Read the model definition and answer for the solid it produces. Units are mm, in the model's axes. A direction names the side the tool comes from. Round coordinates to 2 decimals unless told otherwise and drop trailing zeros. Write each loop counter-clockwise with the first axis right and the second up, starting at its lowest first coordinate (ties: lowest second). Pieces come first, ordered by that corner, then holes. Notation, with made-up numbers: (14.5, 27) -> (31.5, 27) arc R31 ccw to (31.5, 60) -> close; hole circle Ø5 at (7, 60). An arc over 180 degrees is marked (long way). Return JSON: item names as keys, results as strings. Group by question number.
(1) A cutting plane is placed at A-A on z = 15. Give the vertices of the cut face in (x, y), then the cut area to 3 significant figures.
(2) Straight lines are drawn through the part: line 1 (Z direction, x = 8, y = 1.25); line 2 (X direction, y = 2.25, z = 13.5); line 3 (Y direction, x = 4.75, z = 14.5). For each, find the intervals that lie inside material, in ascending order.
(3) A cutting plane is placed at C-C on y = 1. Give the vertices of the cut face in (x, z).
(4) A cutting plane is placed at B-B on z = 5. Give the vertices of the cut face in (x, y), then the cut area to 3 significant figures.
(5) Given pin 1 (3.5 mm diameter, centred on x = 7, z = 14.5, fed in from +Y); pin 2 (3.5 mm diameter, centred on x = 9.5, z = 14.5, fed in from -Y); pin 3 (2 mm diameter, centred on x = 9.5, z = 4.5, fed in from -Y), each flat-ended and moving along its own axis, determine where each tip first touches the part or whether it passes through.
(6) A cutting plane is placed at D-D on x = 1.5. Give the vertices of the cut face in (y, z) (3 decimals).
(7) The mould has two halves that part along X. Classify faces 1 (the flat face through (6.9, 4.5, -8.5)), 2 (the flat face through (6.9, 2, -6.5)), 3 (the flat face through (4, 3.5, -7.7)): released by +X, released by -X, zero draft, split by the parting line, or undercut.
(8) For faces 4 (the flat face through (9, 1, -5)), 5 (the flat face through (7, 1, -6)), 6 (the flat face through (6.9, 4.5, -6.5)), 7 (the flat face through (1.2, 3, 17)), 8 (the flat face through (7, 1.5, 17)), determine the directions among +Z, -Z, +X, -X, +Y, -Y from which every point of the face is accessible in a straight line to the end or side of a thin tool.
Autodesk Fusion 360 part; units mm, degrees
sketch "草图1" plane through (0, 0, 0) normal (0, 1, 0) x (1, 0, 0)
  line L0 (0, 0) -> (14, 0)
  line L1 (14, 0) -> (14, -11)
  line L2 (14, -11) -> (0, -11)
  line L3 (0, -11) -> (0, 0)
  line L4 (7, -11) -> (7, 8) construction
  line L5 (7, 5) -> (10, 5)
  line L6 (7, 5) -> (4, 5)
  line L7 (0, 0) -> (4, 5)
  line L8 (14, 0) -> (10, 5)
  dimension "d1" = 14
  dimension "d2" = 11
  dimension "d3" = 3
  dimension "d4" = 3
  dimension "d5" = 5
extrude "拉伸1" add sketch "草图1" along normal blind 7
sketch "草图2" plane through (0, 0, 11) normal (0, 0, 1) x (-1, 0, 0)
  line L0 (0, 0) -> (-14, 0)
  line L1 (-14, 0) -> (-14, -7)
  line L2 (-14, -7) -> (0, -7)
  line L3 (0, -7) -> (0, 0)
  line L4 (-1, -5.5) -> (-13, -5.5)
  line L5 (-13, -5.5) -> (-13, -1.5)
  line L6 (-13, -1.5) -> (-1, -1.5)
  line L7 (-1, -1.5) -> (-1, -5.5)
  line L8 (-1.2, -1.7) -> (-1.2, -5.3)
  line L9 (-1.2, -5.3) -> (-12.8, -5.3)
  line L10 (-12.8, -5.3) -> (-12.8, -1.7)
  line L11 (-12.8, -1.7) -> (-1.2, -1.7)
  line L12 (-1.2, -3.5) -> (-12.8, -3.5)
  dimension "d8" = 12
  dimension "d9" = 4
  dimension "d10" = 1.5
  dimension "d11" = 1
  dimension "d12" = 0.2
extrude "拉伸2" add sketch "草图2" along normal blind 12 contours L4 L5 L6 L7
extrude "拉伸3" add sketch "草图2" along normal blind 11 contours L8 L9 L10 L12
sketch "草图3" plane through (0, 0, 0) normal (0, -1, 0) x (1, 0, 0)
  line L0 (14, 0) -> (14, 11)
  line L1 (14, 11) -> (0, 11)
  line L2 (0, 11) -> (0, 0)
  line L3 (0, 0) -> (4, -5)
  line L4 (4, -5) -> (10, -5)
  line L5 (10, -5) -> (14, 0)
  line L6 (2, 9) -> (12, 9)
  line L7 (12, 9) -> (12, 0)
  line L8 (12, 0) -> (2, 0)
  line L9 (2, 0) -> (2, 9)
extrude "拉伸4" cut sketch "草图3" against normal blind 0.2 contours L6 L7 L8 L9
sketch "草图4" plane through (0, 7, 0) normal (0, 1, 0) x (-1, 0, 0)
  line L0 (-14, 11) -> (-14, 0)
  line L1 (-14, 0) -> (-10, -5)
  line L2 (-10, -5) -> (-4, -5)
  line L3 (-4, -5) -> (0, 0)
  line L4 (0, 0) -> (0, 11)
  line L5 (0, 11) -> (-14, 11)
  line L6 (-12, 9) -> (-2, 9)
  line L7 (-2, 9) -> (-2, 0)
  line L8 (-2, 0) -> (-12, 0)
  line L9 (-12, 0) -> (-12, 9)
extrude "拉伸5" cut sketch "草图4" against normal blind 0.2 contours L6 L7 L8 L9
sketch "草图5" plane through (0, 1.5, 0) normal (0, -1, 0) x (1, 0, 0)
  line L0 (1, 11) -> (13, 11)
  line L1 (13, 11) -> (13, 23)
  line L2 (13, 23) -> (1, 23)
  line L3 (1, 23) -> (1, 11)
  line L4 (7, 11) -> (7, 23) construction
  line L5 (2.5, 20) -> (5.5, 20)
  line L6 (5.5, 20) -> (5.5, 18)
  line L7 (5.5, 18) -> (2.5, 18)
  line L8 (2.5, 18) -> (2.5, 20)
  line L9 (11.5, 20) -> (8.5, 20)
  line L10 (11.5, 18) -> (11.5, 20)
  line L11 (8.5, 18) -> (11.5, 18)
  line L12 (8.5, 20) -> (8.5, 18)
  dimension "d21" = 1.5
extrude "拉伸6" cut sketch "草图5" against normal up to surface (0.2 mm away) contours L5 L6 L7 L8 | L9 L10 L11 L12
sketch "草图6" plane through (0, 0, -5) normal (0, 0, -1) x (1, 0, 0)
  line L0 (10, 0) -> (4, 0)
  line L1 (4, 0) -> (4, -7)
  line L2 (4, -7) -> (10, -7)
  line L3 (10, -7) -> (10, 0)
  circle A0 centre (6.9717, -3.5) radius 3
  dimension "d24" = 6
extrude "拉伸7" add sketch "草图6" along normal blind 5.5 contours L1 A0 picked at (7.5942, -2.8884)
sketch "草图7" plane through (0, 0, 0) normal (0, 1, 0) x (1, 0, 0)
  line L0 (4, 6) -> (10, 6)
  line L1 (10, 6) -> (10, 7)
  line L2 (10, 7) -> (4, 7)
  line L3 (4, 7) -> (4, 6)
  line L4 (4, 8) -> (10, 8)
  line L5 (10, 8) -> (10, 9)
  line L6 (10, 9) -> (4, 9)
  line L7 (4, 9) -> (4, 8)
extrude "拉伸8" cut sketch "草图7" along normal blind 2
extrude "拉伸9" cut 2 faces at (6.1056, 2, -6.3333) (6.1056, 2, -8.3333) along direction (0, 1, 0) blind 2 from surface at 2.5
Checks:
{
 "1": {"outline": "(1, 1.5) -> (13, 1.5) -> (13, 5.5) -> (1, 5.5) -> close; hole (1.2, 1.7) -> (12.8, 1.7) -> (12.8, 3.5) -> (1.2, 3.5) -> close", "area": "27.1 mm^2"},
 "2": {"line 1": "z = -10.5 to -9, -8 to -7, -6 to 11", "line 2": "x = 1 to 1.2, 12.8 to 13", "line 3": "y = 1.5 to 1.7, 3.5 to 5.5"},
 "3": {"outline": "(0, 0) -> (4, -5) -> (5.31, -5) -> (5.31, -6) -> (8.63, -6) -> (8.63, -5) -> (10, -5) -> (14, 0) -> (14, 11) -> (0, 11) -> close; (5.31, -10.5) -> (8.63, -10.5) -> (8.63, -9) -> (5.31, -9) -> close; (5.31, -8) -> (8.63, -8) -> (8.63, -7) -> (5.31, -7) -> close"},
 "4": {"outline": "(0, 0) -> (2, 0) -> (2, 0.2) -> (12, 0.2) -> (12, 0) -> (14, 0) -> (14, 7) -> (12, 7) -> (12, 6.8) -> (2, 6.8) -> (2, 7) -> (0, 7) -> close", "area": "94.0 mm^2"},
 "5": {"pin 1": "stops at y = 5.5", "pin 2": "stops at y = 1.5", "pin 3": "stops at y = 0.2"},
 "6": {"outline": "(0, -1.875) -> (7, -1.875) -> (7, 11) -> (5.5, 11) -> (5.5, 23) -> (5.3, 23) -> (5.3, 22) -> (3.5, 22) -> (3.5, 11) -> (1.7, 11) -> (1.7, 23) -> (1.5, 23) -> (1.5, 11) -> (0, 11) -> close"},
 "7": {"face 1": "undercut", "face 2": "zero draft", "face 3": "released by -X"},
 "8": {"face 4": "-Z", "face 5": "+X, -X, -Y", "face 6": "+Y", "face 7": "+Z", "face 8": "+Z, +X, -X, -Y"}
}
